Geometry check sheet. Reference: the model listing, model coordinates, mm. Face numbers are marked on the shaded views. A direction names the side the tool comes from. Round coordinates to 2 decimals unless told otherwise and drop trailing zeros. Loops run counter-clockwise (first coordinate to the right, second up) from the corner with the lowest first, then second, coordinate; pieces in that order, holes last. Notation, with made-up numbers: (79.25, 30) - (119.25, 30) arc R20 cw to (119.25, 44) - close; hole circle Ø10 at (-31.5, -10). An arc over 180 degrees is marked (long way). Answer in a Markdown table with one row per item. Add a question column.
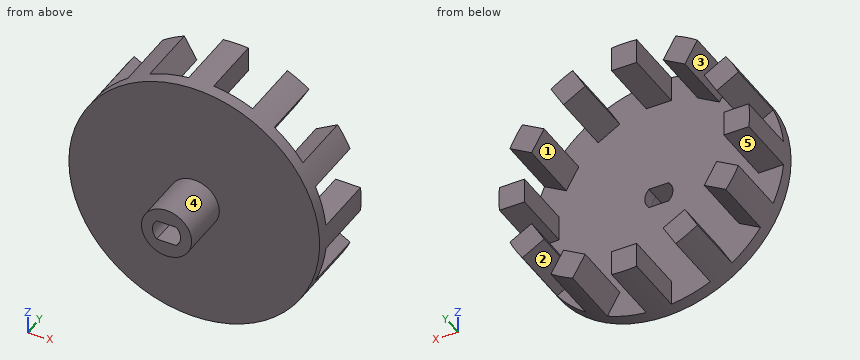
Autodesk Fusion 360 part; units mm, degrees
sketch "Sketch1" plane through (0, 0, 0) normal (0, 1, 0) x (1, 0, 0)
  circle A0 centre (0, 0) radius 2.805
  line L0 (-2.805, 2) -> (2.805, 2)
  line L1 (2.805, 2) -> (2.805, -2)
  line L2 (2.805, -2) -> (-2.805, -2)
  line L3 (-2.805, -2) -> (-2.805, 2)
  line L4 (0, 2) -> (0, 0) construction
  line L5 (0, 0) -> (0, -2) construction
  circle A1 centre (0, 0) radius 5
  dimension "d1" = 5.61
  dimension "d2" = 2
  dimension "d3" = 10
extrude "Extrude1" add sketch "Sketch1" along normal blind 10 contours A0 L1 L2 | A0 L0 L1 | A0 L0 | A0 L2 | A0 L0 L3 | A0 L2 L3 | A1
sketch "Sketch2" plane through (0, 10, 0) normal (0, 1, 0) x (-1, 0, 0)
  arc A0 (1.9667, -2) -> (1.9667, 2) centre (0, 0) ccw
  line L0 (1.9667, -2) -> (-1.9667, -2)
  arc A1 (-1.9667, 2) -> (-1.9667, -2) centre (0, 0) ccw
  line L1 (-1.9667, 2) -> (1.9667, 2)
  circle A2 centre (0, 0) radius 5
  circle A3 centre (0, 0) radius 25
  line L2 (-2.5, -24.8747) -> (-2.5, -19.8747)
  line L3 (-2.5, -19.8747) -> (2.5, -19.8747)
  line L4 (2.5, -19.8747) -> (2.5, -24.8747)
  line L5 (12.1024, -15.962) -> (14.6024, -20.2921)
  line L6 (7.7723, -18.462) -> (12.1024, -15.962)
  line L7 (10.2723, -22.7921) -> (7.7723, -18.462)
  line L8 (18.462, -7.7723) -> (22.7921, -10.2723)
  line L9 (15.962, -12.1024) -> (18.462, -7.7723)
  line L10 (20.2921, -14.6024) -> (15.962, -12.1024)
  line L11 (19.8747, 2.5) -> (24.8747, 2.5)
  line L12 (19.8747, -2.5) -> (19.8747, 2.5)
  line L13 (24.8747, -2.5) -> (19.8747, -2.5)
  line L14 (15.962, 12.1024) -> (20.2921, 14.6024)
  line L15 (18.462, 7.7723) -> (15.962, 12.1024)
  line L16 (22.7921, 10.2723) -> (18.462, 7.7723)
  line L17 (7.7723, 18.462) -> (10.2723, 22.7921)
  line L18 (12.1024, 15.962) -> (7.7723, 18.462)
  line L19 (14.6024, 20.2921) -> (12.1024, 15.962)
  line L20 (-2.5, 19.8747) -> (-2.5, 24.8747)
  line L21 (2.5, 19.8747) -> (-2.5, 19.8747)
  line L22 (2.5, 24.8747) -> (2.5, 19.8747)
  line L23 (-12.1024, 15.962) -> (-14.6024, 20.2921)
  line L24 (-7.7723, 18.462) -> (-12.1024, 15.962)
  line L25 (-10.2723, 22.7921) -> (-7.7723, 18.462)
  line L26 (-18.462, 7.7723) -> (-22.7921, 10.2723)
  line L27 (-15.962, 12.1024) -> (-18.462, 7.7723)
  line L28 (-20.2921, 14.6024) -> (-15.962, 12.1024)
  line L29 (-19.8747, -2.5) -> (-24.8747, -2.5)
  line L30 (-19.8747, 2.5) -> (-19.8747, -2.5)
  line L31 (-24.8747, 2.5) -> (-19.8747, 2.5)
  line L32 (-15.962, -12.1024) -> (-20.2921, -14.6024)
  line L33 (-18.462, -7.7723) -> (-15.962, -12.1024)
  line L34 (-22.7921, -10.2723) -> (-18.462, -7.7723)
  line L35 (-7.7723, -18.462) -> (-10.2723, -22.7921)
  line L36 (-12.1024, -15.962) -> (-7.7723, -18.462)
  line L37 (-14.6024, -20.2921) -> (-12.1024, -15.962)
  dimension "d6" = 50
  dimension "d7" = 5
  dimension "d9" = 360
extrude "Extrude2" add sketch "Sketch2" along normal blind 2.5 contours A2 | A3 L2 L3 L4 L5 L6 L7 L8 L9 L10 L11 L12 L13 L14 L15 L16 L17 L18 L19 L20 L21 L22 L23 L24 L25 L26 L27 L28 L29 L30 L31 L32 L33 L34 L35 L36 L37
extrude "Extrude3" add sketch "Sketch2" along normal blind 15 contours A3 L11 L12 L13 | A3 L14 L15 L16 | A3 L8 L9 L10 | A3 L17 L18 L19 | A3 L5 L6 L7 | A3 L20 L21 L22 | A3 L2 L3 L4 | A3 L23 L24 L25 | A3 L35 L36 L37 | A3 L26 L27 L28 | A3 L32 L33 L34 | A3 L29 L30 L31
equation "d1 = ( 5.5 * 1.02 ) * 1 mm"
Q1. Depth check by flat-ended pin: P1, Ø15, axis at x = -9.5, z = 5.5, coming from the -Y side; P2, Ø1.5, axis at x = 23, y = 21.5, coming from the +Z side; P3, Ø12, axis at x = -11.5, z = -18.5, coming from the -Y side; P4, Ø2, axis at x = 0.5, y = 8.5, coming from the -Z side. Enter the tip coordinate at first touch or a pass-through.
Q2. Cross-section at A-A, the plane x = 0. Enter the section's corners in (y, z).
Q3. Cross-section at B-B, the plane z = 0. Enter the section's corners in (x, y) (3 decimals).
Q4. Set-up check for the marked faces 1, 2, 3, 4 and 5: record each of +Z, -Z, +X, -X, +Y, -Y from which the full face is reachable in a straight line by a thin tool's end or side.
Q5. Scan lines: line 1 (Y direction, x = 15, z = 8); line 2 (Z direction, x = -11.5, y = 15.5); line 3 (Y direction, x = -16.5, z = 12). Record each from-to range of solid material in increasing order. Write a range as from..to.
Q6. Cross-section at D-D, the plane z = 7. Enter the section's corners in (x, y).
Q7. Cross-section at C-C, the plane y = 4.25. Enter the section's corners in (x, z) (3 decimals), plus the area to 3 significant figures.
Check sheet entries:
| question | item | result |
|---|---|---|
| 1 | P1 | y = 0 |
| 1 | P2 | z = 11.4 |
| 1 | P3 | y = 10 |
| 1 | P4 | z = -5 |
| 2 | outline | (0, -5) - (10, -5) - (10, -25) - (25, -25) - (25, -19.87) - (12.5, -19.87) - (12.5, -2) - (0, -2) - close; (0, 2) - (12.5, 2) - (12.5, 19.87) - (25, 19.87) - (25, 25) - (10, 25) - (10, 5) - (0, 5) - close |
| 3 | outline | (-25, 10) - (-5, 10) - (-5, 0) - (-2.805, 0) - (-2.805, 12.5) - (-19.875, 12.5) - (-19.875, 25) - (-25, 25) - close; (2.805, 0) - (5, 0) - (5, 10) - (25, 10) - (25, 25) - (19.875, 25) - (19.875, 12.5) - (2.805, 12.5) - close |
| 4 | face 1 | +Y |
| 4 | face 2 | -Z, +Y |
| 4 | face 3 | -X, +Y |
| 4 | face 4 | -Y |
| 4 | face 5 | +X, -X, +Y |
| 5 | line 1 | 10..12.5 |
| 5 | line 2 | -22.2..-16.31, 16.31..22.2 |
| 5 | line 3 | 10..25 |
| 6 | outline | (-24, 10) - (24, 10) - (24, 12.5) - (-24, 12.5) - close |
| 7 | outline | circle Ø10 at (0, 0); hole (-1.967, -2) - (1.967, -2) arc R2.805 ccw to (1.967, 2) - (-1.967, 2) arc R2.805 ccw to start |
| 7 | area | 58.2 mm² |
